Job drawing, mm, ordinate dimensions from the low corner. One solid piece. A direction names the side the tool comes from. Give positions to 0.01 mm unless a question says otherwise; leave off trailing zeros. Loops run counter-clockwise (first coordinate to the right, second up) from the corner with the lowest first, then second, coordinate; pieces in that order, holes last. Notation, with made-up numbers: M 59.5,75.25 L 68.5,75.25 A20 cw 68.5,111.25 Z; hole C 8,-31 d8. An arc over 180 degrees is marked long. Put each result on its own line as item: value.
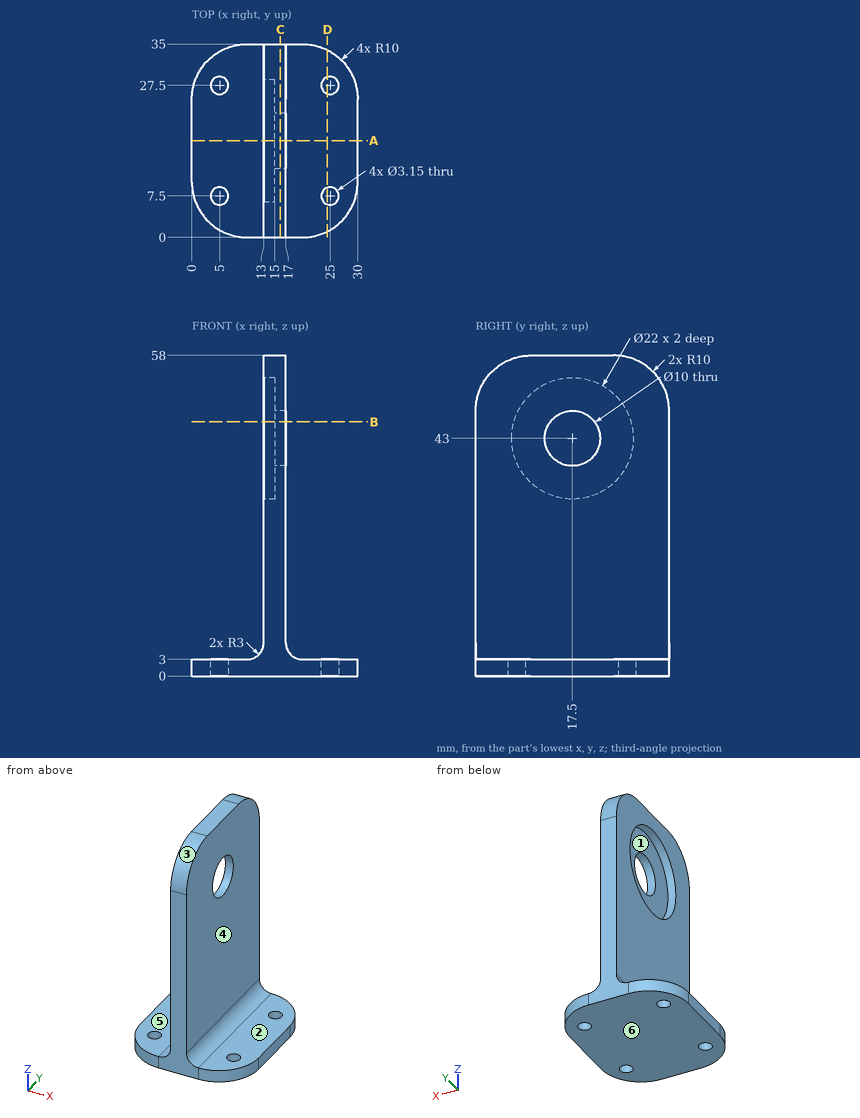
Q1. Tool access for the marked faces 4, 5 and 6: list every direction of +Z, -Z, +X, -X, +Y, -Y with a clear straight run to the whole face (end or side of a thin tool).
Here are the results:
face 4: +Z, +X, +Y, -Y
face 5: +Z, -X, +Y, -Y
face 6: -Z, +X, -X, +Y, -Y
Q2. Slice it at C-C (x = 16). List the corners of the cut face in (y, z).
Here are the results:
outline: M 0,0 L 35,0 L 35,48 A10 ccw 25,58 L 10,58 A10 ccw 0,48 Z; hole C 17.5,43 d10
Q3. Drop flat-ended pins along their axis: pin 1 Ø1.9 at (x, y) = (5, 7.5) entering from +Z; pin 2 Ø8 at (x, y) = (4, 19.5) entering from +Z; pin 3 Ø10 at (y, z) = (4.5, 45.5) entering from -X; pin 4 Ø4 at (y, z) = (16, 6.5) entering from +X. Give the stop position or say it passes through.
Here are the results:
pin 1: through
pin 2: z = 3
pin 3: x = 13
pin 4: x = 17.4
Q4. Slice it at A-A (y = 17.5). List the corners of the cut face in (x, z).
Here are the results:
outline: M 0,0 L 30,0 L 30,3 L 20,3 A3 cw 17,6 L 17,38 L 15,38 L 15,32 L 13,32 L 13,6 A3 cw 10,3 L 0,3 Z; M 13,54 L 15,54 L 15,48 L 17,48 L 17,58 L 13,58 Z
Q5. Slice it at D-D (x = 24.5). List the corners of the cut face in (y, z), and give its area (3 significant figures).
Here are the results:
outline: M 1.07,0 L 6.01,0 L 6.01,3 L 1.07,3 Z; M 8.99,0 L 26.01,0 L 26.01,3 L 8.99,3 Z; M 28.99,0 L 33.93,0 L 33.93,3 L 28.99,3 Z
area: 80.7 mm²
Q6. Mould opens along Y. For the marked faces 1, 2 and 3 say: pulls with the +Y half, pulls with the -Y half, needs draft (parallel to the pull), parting line crosses it, or undercut.
Here are the results:
face 1: undercut
face 2: needs draft
face 3: pulls with the -Y half
Q7. Probe line 1 (Z direction, x = 15.5, y = 17.5); line 2 (Y direction, x = 25, z = 1) (3 decimals); line 3 (Z direction, x = 25, y = 21.5). List the from-to ranges inside material, lowest first. Write a range as from..to.
Here are the results:
line 1: 0..38, 48..58
line 2: 1.34..5.925, 9.075..25.925, 29.075..33.66
line 3: 0..3
Q8. Slice it at B-B (z = 46). List the corners of the cut face in (x, y), and give its area (3 significant figures).
Here are the results:
outline: M 13,0 L 17,0 L 17,13.5 L 15,13.5 L 15,6.92 L 13,6.92 Z; M 13,28.08 L 15,28.08 L 15,21.5 L 17,21.5 L 17,35 L 13,35 Z
area: 81.7 mm²
